Can you work these out from the model? Positions are in its coordinate system, mm. Face numbers are marked on the shaded views. A direction names the side the tool comes from. Give positions to 0.01 mm unless a question says otherwise; leave off trailing zeros. Loops run counter-clockwise (first coordinate to the right, second up) from the corner with the lowest first, then second, coordinate; pieces in that order, holes last. Notation, with made-up numbers: M 65,80 L 95,80 A18 ccw 95,85 Z; hole C 53.5,14 d3. An arc over 180 degrees is marked long. Answer as a JSON object with one key per item and string values.
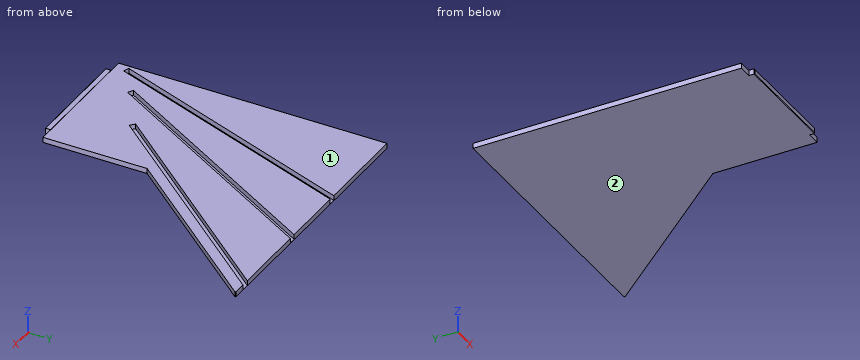
```python
from build123d import *

# Parameters (mm, degrees)
BOSS_EXTRUDE1_DEPTH = 1.9
BOSS_EXTRUDE5_DEPTH = 0.1
SKETCH6_W           = 40
SKETCH6_H           = 2
BOSS_EXTRUDE6_DEPTH = 0.1
CHAMFER2_SIZE       = 0.2


with BuildPart() as part:
    # Sketch1 → Boss-Extrude1 (new body)
    with BuildSketch(Plane.XY):
        Polygon((-36.312345137, -37.152540378), (-38.217601025, -36.052540378), (11.464856327, 50), (-12.432381024, 50), (-46.771329023, -44.345484236), (-48.838652789, -43.593039921), (-14.773572123, 50), (-50, 50), (-50, -48), (-45, -48), (-45, -50), (-5, -50), (-5, -48), (0, -48), (0, -10), (50, 49.58767963), (50, 50), (45.345911136, 50), (-19.526148963, -27.311510683), (-21.211446738, -25.897377941), (42.474015099, 50), (14.005197511, 50), align=None)
    extrude(amount=BOSS_EXTRUDE1_DEPTH)

    # Sketch2 → Boss-Extrude5 (add)
    with BuildSketch(Plane(origin=(0, 0, 0), x_dir=(-1, 0, 0), z_dir=(0, 0, -1))):
        Polygon((-45.345911136, 50), (-42.474015099, 50), (21.211446738, -25.897377941), (19.526148963, -27.311510683), align=None)
        Polygon((-14.005197511, 50), (36.312345137, -37.152540378), (38.217601025, -36.052540378), (-11.464856327, 50), align=None)
        Polygon((12.432381024, 50), (14.773572123, 50), (48.838652789, -43.593039921), (46.771329023, -44.345484236), align=None)
    extrude(amount=-BOSS_EXTRUDE5_DEPTH)

    # Sketch6 → Boss-Extrude6 (add)
    with BuildSketch(Plane.XY.offset(1.9)):
        with Locations((-25, -49)):
            Rectangle(SKETCH6_W, SKETCH6_H)
    extrude(amount=BOSS_EXTRUDE6_DEPTH)

    # Chamfer2
    chamfer2_edges = [part.edges().sort_by_distance(p)[0] for p in [
        (-25, -50, 2),
        (-25, -50, 0),
        (-5, -50, 1),
        (-45, -50, 1),
    ]]
    chamfer(chamfer2_edges, length=CHAMFER2_SIZE)


solid = part.part
```
1) Suppose I cut it at D-D, the plane y = 3. Write out the boundary of the cut face in (x, z).
Answer list:
{"outline": "M -50,0 L 10.91,0 L 10.91,1.9 L 5.91,1.9 L 5.91,0.1 L 3.04,0.1 L 3.04,1.9 L -13.13,1.9 L -13.13,0.1 L -15.67,0.1 L -15.67,1.9 L -29.54,1.9 L -29.54,0.1 L -31.88,0.1 L -31.88,1.9 L -50,1.9 Z"}
2) Suppose I cut it at C-C, the plane x = 31. Write out the boundary of the cut face in (y, z).
Answer list:
{"outline": "M 26.94,0 L 50,0 L 50,1.9 L 36.33,1.9 L 36.33,0.1 L 32.9,0.1 L 32.9,1.9 L 26.94,1.9 Z"}
3) For the marked faces 1 and 2, which set-ups out of +Z, -Z, +X, -X, +Y, -Y let a thin tool reach every point of the face, with its end or its side?
Answer list:
{"face 1": "+Z, +X, -X, +Y", "face 2": "-Z, +X, -X, +Y, -Y"}
4) Suppose I cut it at A-A, the plane z = 1.4. Write out the boundary of the cut face in (x, y), and give its area (3 significant figures).
Answer list:
{"outline": "M -50,-48 L -45,-48 L -45,-49.8 L -44.8,-50 L -5.2,-50 L -5,-49.8 L -5,-48 L 0,-48 L 0,-10 L 50,49.59 L 50,50 L 45.35,50 L -19.53,-27.31 L -21.21,-25.9 L 42.47,50 L 14.01,50 L -36.31,-37.15 L -38.22,-36.05 L 11.46,50 L -12.43,50 L -46.77,-44.35 L -48.84,-43.59 L -14.77,50 L -50,50 Z", "area": "5,830 mm^2"}
5) Will these pins go through, and if not, where does the flat tip stop? pin 1 Ø1 at (y, z) = (-28, 0.5) entering from +X; pin 2 Ø18 at (x, y) = (-22, 11) entering from +Z; pin 3 Ø1 at (y, z) = (9.5, 1) entering from +X; pin 4 Ø1.5 at (x, y) = (21.5, 14) entering from -Z.
Answer list:
{"pin 1": "x = 0", "pin 2": "z = 1.9", "pin 3": "x = 16.78", "pin 4": "through"}
6) Please list where these lines run through material, in increasing order: line 1 along X through (y, z) = (38.5, 1.65); line 2 along X through (y, z) = (45, 1.3); line 3 along X through (y, z) = (-33.5, 1.3). Write a range as from..to.
Answer list:
{"line 1": "-50..-18.96, -16.62..4.83, 7.37..32.82, 35.7..40.7", "line 2": "-50..-16.59, -14.25..8.58, 11.12..38.28, 41.15..46.15", "line 3": "-50..-45.17, -42.82..-36.74, -34.2..0"}
7) Suppose I cut it at B-B, the plane y = 24. Write out the boundary of the cut face in (x, z), and give its area (3 significant figures).
Answer list:
{"outline": "M -50,0 L 28.53,0 L 28.53,1.9 L 23.53,1.9 L 23.53,0.1 L 20.66,0.1 L 20.66,1.9 L -1.01,1.9 L -1.01,0.1 L -3.55,0.1 L -3.55,1.9 L -21.9,1.9 L -21.9,0.1 L -24.24,0.1 L -24.24,1.9 L -50,1.9 Z", "area": "135 mm^2"}
